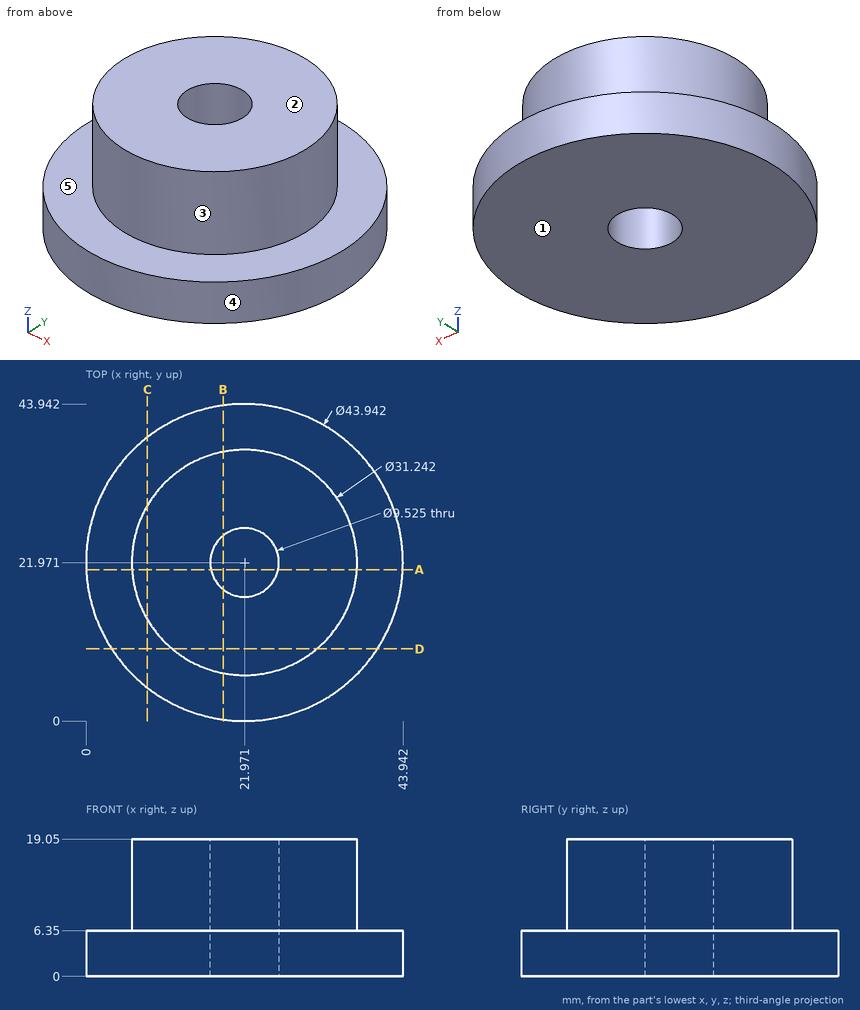
For this review, use the dimensioned drawing (mm, ordinates from the lowest corner) and the shaded views. A direction names the side the tool comes from. Give positions to 0.01 mm unless a question says otherwise; leave off trailing zeros. Write each loop counter-clockwise with the first axis right and the second up, starting at its lowest first coordinate (ties: lowest second). Pieces come first, ordered by that corner, then holes. Notation, with made-up numbers: M 89,-19 L 144,-19 A28 ccw 144,11 Z; hole C 83,71 d4. An arc over 180 degrees is marked long. Write item = value, one per line. Start each with the question number.
Q1. We need section A-A (y = 21). State the section outline as (x, z) points.
Q2. For line 1 (Y direction, x = 19, z = 3.5); line 2 (Y direction, x = 25, z = 1.25); line 3 (Z direction, x = 27.5, y = 3.5), list the stretches that pass through material, from the lowest coordinate up.
Q3. We need section B-B (x = 19). State the section outline as (y, z) points.
Q4. Machinability: for the marked faces 4 and 5, which of the approach directions +Z, -Z, +X, -X, +Y, -Y give a long, thin tool a straight path to every point of the face, cutting with its end or side? Answer none if there is none.
Q5. Clearance check with flat-ended pins moving along their axes: pin 1 (3 mm diameter, centred on y = 25, z = 4.5, fed in from -X); pin 2 (5 mm diameter, centred on y = 5, z = 14.5, fed in from -X); pin 3 (7.5 mm diameter, centred on x = 21.971, y = 21.971, fed in from -Z) (3 decimals); pin 4 (1.5 mm diameter, centred on y = 13, z = 17, fed in from -X). State where each tip first meets the part, or that it passes through.
Q6. We need section C-C (x = 8.5). State the section outline as (y, z) points.
Q7. We need section D-D (y = 10). State the section outline as (x, z) points.
Q8. Mouldability with a two-part tool opening along Z and no side actions: class the marked faces 1, 2 and 3 as released by +Z, released by -Z, zero draft, split by the parting line, or undercut.
Result set:
q1.outline = M 0.02,0 L 17.31,0 L 17.31,19.05 L 6.38,19.05 L 6.38,6.35 L 0.02,6.35 Z; M 26.63,0 L 43.92,0 L 43.92,6.35 L 37.56,6.35 L 37.56,19.05 L 26.63,19.05 Z
q2.line_1 = 0.2 to 18.25, 25.69 to 43.74
q2.line_2 = 0.21 to 18.3, 25.65 to 43.73
q2.line_3 = 0 to 6.35
q3.outline = M 0.2,0 L 18.25,0 L 18.25,19.05 L 6.64,19.05 L 6.64,6.35 L 0.2,6.35 Z; M 25.69,0 L 43.74,0 L 43.74,6.35 L 37.31,6.35 L 37.31,19.05 L 25.69,19.05 Z
q4.face_4 = +Z, -Z
q4.face_5 = +Z
q5.pin_1 = 0.05
q5.pin_2 = 16.09
q5.pin_3 = through
q5.pin_4 = 8.69
q6.outline = M 4.61,0 L 39.33,0 L 39.33,6.35 L 29.88,6.35 L 29.88,19.05 L 14.06,19.05 L 14.06,6.35 L 4.61,6.35 Z
q7.outline = M 3.55,0 L 40.39,0 L 40.39,6.35 L 32.01,6.35 L 32.01,19.05 L 11.94,19.05 L 11.94,6.35 L 3.55,6.35 Z
q8.face_1 = released by -Z
q8.face_2 = released by +Z
q8.face_3 = zero draft
